```python
from build123d import *

# Parameters (mm, degrees)
SKETCH1_W           = 110
SKETCH1_H           = 50
SKETCH1_R           = 1.75
BOSS_EXTRUDE1_DEPTH = 8
SKETCH2_W           = 43
SKETCH2_H           = 50
CUT_EXTRUDE1_DEPTH  = 3
SKETCH3_R           = 3
CUT_EXTRUDE2_DEPTH  = 5
FILLET1_R           = 10
FILLET2_R           = 10
SKETCH4_R           = 1
CUT_EXTRUDE3_DEPTH  = 122.095004026


with BuildPart() as part:
    # Sketch1 → Boss-Extrude1 (new body)
    with BuildSketch(Plane(origin=(0, 0, 0), x_dir=(1, 0, 0), z_dir=(0, 1, 0))):
        with Locations((55, 25)):
            Rectangle(SKETCH1_W, SKETCH1_H)
        with Locations(Location((50, 40, 0), (0, 0, 270))):
            Circle(SKETCH1_R, mode=Mode.SUBTRACT)
        with Locations(Location((50, 10, 0), (0, 0, 270))):
            Circle(SKETCH1_R, mode=Mode.SUBTRACT)
    extrude(amount=BOSS_EXTRUDE1_DEPTH)

    # Sketch2 → Cut-Extrude1 (cut)
    with BuildSketch(Plane.XZ):
        with Locations((21.5, -25)):
            Rectangle(SKETCH2_W, SKETCH2_H)
    extrude(amount=-CUT_EXTRUDE1_DEPTH, mode=Mode.SUBTRACT)

    # Sketch3 → Cut-Extrude2 (cut)
    with BuildSketch(Plane(origin=(0, 8, 0), x_dir=(1, 0, 0), z_dir=(0, 1, 0))):
        with Locations(Location((50, 40, 0), (0, 0, 270))):
            Circle(SKETCH3_R)
        with Locations(Location((50, 10, 0), (0, 0, 270))):
            Circle(SKETCH3_R)
    extrude(amount=-CUT_EXTRUDE2_DEPTH, mode=Mode.SUBTRACT)

    # Fillet1
    # the kernel refuses this fillet: 10 mm, written as the material it adds along each edge
    with BuildSketch(Plane(origin=(43, 3, 0), x_dir=(-1, 0, 0), z_dir=(0, 0, -1))) as fillet1_piece_1:
        with BuildLine():
            CenterArc((7.141428429, -10), FILLET1_R, 90, 45.572995999)
            Line((0, -3), (-0.142828569, -2.86))
            ThreePointArc((-0.142828569, -2.86), (-0.2, -1.5), (-0.2, 0))
            Line((-0.2, 0), (0, 0.2))
            Line((0, 0.2), (7.141428429, 0.2))
            Line((7.141428429, 0.2), (7.141428429, 0))
        make_face()
    extrude(amount=50)

    # Fillet2
    fillet2_edges = [part.edges().sort_by_distance(p)[0] for p in [
        (0, 5.5, -50),
        (110, 4, -50),
        (110, 4, 0),
        (0, 5.5, 0),
    ]]
    fillet(fillet2_edges, radius=FILLET2_R)

    # Sketch4 → Cut-Extrude3 (cut, through all)
    with BuildSketch(Plane(origin=(0, 8, 0), x_dir=(1, 0, 0), z_dir=(0, 1, 0))):
        with Locations(Location((5, 25, 0), (0, 0, 270))):
            Circle(SKETCH4_R)
        with Locations(Location((105, 25, 0), (0, 0, 270))):
            Circle(SKETCH4_R)
    extrude(amount=-CUT_EXTRUDE3_DEPTH, mode=Mode.SUBTRACT)


solid = part.part
```
Geometry: final body of the model. Coordinates: model frame, mm. A direction names the side the tool comes from. Coordinates: 2 decimals unless noted, no trailing zeros. Order: outer loops, then holes, each group sorted by start corner. A loop starts at its lowest first (then second) coordinate and runs counter-clockwise, first axis right, second up. Notation, with made-up numbers: (-6, -34) -> (6, -34) arc R21 ccw to (6, -21) -> close; hole circle Ø2 at (79, 71.5). An arc over 180 degrees is marked (long way). Answer in a Markdown table with one row per item.
Item 1: Draft query along X for faces 4 (the cylindrical face through (104, 4, -25)), 5 (the flat face through (54, 4, 0)), 6 (the flat face through (110, 4, -25)). Return one class per face: released by +X, released by -X, zero draft, split by the parting line, or undercut.
Return value:
| item | result |
|---|---|
| face 4 | undercut |
| face 5 | zero draft |
| face 6 | released by +X |
Item 2: Contact query for flat-ended pins moving along their axis: P1, Ø2, axis at x = 50, z = -10, coming from the -Y side; P2, Ø4, axis at x = 50, z = -40, coming from the +Y side; P3, Ø4, axis at y = 6.5, z = -6.5, coming from the +X side. Output: stop coordinate, or through.
Return value:
| item | result |
|---|---|
| P1 | passes through |
| P2 | stops at y = 3 |
| P3 | stops at x = 109.89 |
Item 3: Access query for faces 1 (the cylindrical face through (106.99, 4.06, -47.15)), 2 (the flat face through (48, 3, -40)), 3 (the flat face through (18, 3, -25)). Directions: +Z, -Z, +X, -X, +Y, -Y. A direction counts if a zero-diameter tool reaches every point of the face in a straight line with its end or side. Return the directions, or none.
Return value:
| item | result |
|---|---|
| face 1 | -Z, +X, +Y, -Y |
| face 2 | +Y |
| face 3 | +Z, -Z, -X, -Y |
Item 4: Section D-D on y = 7. Output: boundary loops of the cut face in (x, z), plus the area to 3 significant figures.
Return value:
| item | result |
|---|---|
| outline | (0, -40) arc R10 ccw to (10, -50) -> (100, -50) arc R10 ccw to (110, -40) -> (110, -10) arc R10 ccw to (100, 0) -> (10, 0) arc R10 ccw to (0, -10) -> close; hole circle Ø2 at (5, -25); hole circle Ø6 at (50, -40); hole circle Ø6 at (50, -10); hole circle Ø2 at (105, -25) |
| area | 5,350 mm² |
Item 5: Section C-C on x = 5. Output: boundary loops of the cut face in (y, z).
Return value:
| item | result |
|---|---|
| outline | (3, -48.66) -> (8, -48.66) -> (8, -26) -> (3, -26) -> close; (3, -24) -> (8, -24) -> (8, -1.34) -> (3, -1.34) -> close |
Item 6: Ray query, L1, parallel to Z at x = 50, y = 1.1; L2, parallel to Y at x = 23, z = -45.5; L3, parallel to X at y = 1.2, z = -40. Return the intervals inside material, ascending.
Return value:
| item | result |
|---|---|
| L1 | z = -50 to -41.75, -38.25 to -11.75, -8.25 to 0 |
| L2 | y = 3 to 8 |
| L3 | x = 41.58 to 48.25, 51.75 to 110 |
Item 7: Section A-A on z = -25. Output: boundary loops of the cut face in (x, y).
Return value:
| item | result |
|---|---|
| outline | (0, 3) -> (4, 3) -> (4, 8) -> (0, 8) -> close; (6, 3) -> (35.86, 3) arc R10 cw to (43, 0) -> (104, 0) -> (104, 8) -> (6, 8) -> close; (106, 0) -> (110, 0) -> (110, 8) -> (106, 8) -> close |
Item 8: Section B-B on y = 1.25. Output: boundary loops of the cut face in (x, z), plus the area to 3 significant figures.
Return value:
| item | result |
|---|---|
| outline | (41.51, -50) -> (100, -50) arc R10 ccw to (110, -40) -> (110, -10) arc R10 ccw to (100, 0) -> (41.51, 0) -> close; hole circle Ø3.5 at (50, -40); hole circle Ø3.5 at (50, -10); hole circle Ø2 at (105, -25) |
| area | 3,360 mm² |
